from build123d import *

# Parameters (mm, degrees)
SKETCH1_R           = 2.6
SKETCH1_W           = 352.775
SKETCH1_H           = 95.6
BOSS_EXTRUDE1_DEPTH = 3


with BuildPart() as part:
    # Sketch1 → Boss-Extrude1 (new body)
    with BuildSketch(Plane(origin=(0, 0, 0), x_dir=(1, 0, 0), z_dir=(0, 1, 0))):
        with BuildLine():
            Line((4.973e-06, 108.599998007), (4.973e-06, 4.999998007))
            ThreePointArc((4.973e-06, 4.999998007), (1.464471067, 1.464464101), (5.000004973, -1.993e-06))
            Line((5.000004973, -1.993e-06), (365.775004973, -1.993e-06))
            ThreePointArc((365.775004973, -1.993e-06), (369.310538879, 1.464464101), (370.775004973, 4.999998007))
            Line((370.775004973, 4.999998007), (370.775004973, 108.599998007))
            ThreePointArc((370.775004973, 108.599998007), (369.310538879, 112.135531913), (365.775004973, 113.599998007))
            Line((365.775004973, 113.599998007), (5.000004973, 113.599998007))
            ThreePointArc((5.000004973, 113.599998007), (1.464471067, 112.135531913), (4.973e-06, 108.599998007))
        make_face()
        with Locations(Location((5.500004973, 108.099998007, 0), (0, 0, 270))):
            Circle(SKETCH1_R, mode=Mode.SUBTRACT)
        with Locations(Location((5.500004973, 5.499998007, 0), (0, 0, 270))):
            Circle(SKETCH1_R, mode=Mode.SUBTRACT)
        with Locations(Location((365.275004973, 5.499998007, 0), (0, 0, 270))):
            Circle(SKETCH1_R, mode=Mode.SUBTRACT)
        with Locations(Location((365.275004973, 108.099998007, 0), (0, 0, 270))):
            Circle(SKETCH1_R, mode=Mode.SUBTRACT)
        with Locations(Location((35.387504973, 4.499998007, 0), (0, 0, 270))):
            Circle(SKETCH1_R, mode=Mode.SUBTRACT)
        with Locations(Location((135.387504973, 4.499998007, 0), (0, 0, 270))):
            Circle(SKETCH1_R, mode=Mode.SUBTRACT)
        with Locations(Location((335.387504973, 4.499998007, 0), (0, 0, 270))):
            Circle(SKETCH1_R, mode=Mode.SUBTRACT)
        with Locations(Location((235.387504973, 4.499998007, 0), (0, 0, 270))):
            Circle(SKETCH1_R, mode=Mode.SUBTRACT)
        with Locations(Location((35.387504973, 109.099998007, 0), (0, 0, 270))):
            Circle(SKETCH1_R, mode=Mode.SUBTRACT)
        with Locations(Location((135.387504973, 109.099998007, 0), (0, 0, 270))):
            Circle(SKETCH1_R, mode=Mode.SUBTRACT)
        with Locations(Location((335.387504973, 109.099998007, 0), (0, 0, 270))):
            Circle(SKETCH1_R, mode=Mode.SUBTRACT)
        with Locations(Location((235.387504973, 109.099998007, 0), (0, 0, 270))):
            Circle(SKETCH1_R, mode=Mode.SUBTRACT)
        with Locations((185.387504973, 56.799998007)):
            Rectangle(SKETCH1_W, SKETCH1_H, mode=Mode.SUBTRACT)
    extrude(amount=-BOSS_EXTRUDE1_DEPTH)


solid = part.part
Geometry: final body of the model. Coordinates: model frame, mm. Round coordinates to 2 decimals unless told otherwise and drop trailing zeros. Loops run counter-clockwise (first coordinate to the right, second up) from the corner with the lowest first, then second, coordinate; pieces in that order, holes last.
Q1. Material intervals for L1, parallel to Z at x = 336, y = -0.65; L2, parallel to Z at x = 138.5, y = -2.15; L3, parallel to X at y = -0.85, z = -29.5 (3 decimals), sorted ascending.
Q2. Section A-A on x = 278.5. Return loops of the section in (y, z), plus the area to 3 significant figures.
Q3. Section C-C on y = -0.5. State how many separate pieces and enclosed holes the cut face has, plus the area to 3 significant figures.
Q4. Section B-B on z = -31. Return loops of the section in (x, y) (3 decimals).
Q5. Pin query (flat end, axial travel): P1, Ø7, axis at x = 235.39, z = -109.1, coming from the +Y side; P2, Ø4, axis at x = 5.5, z = -108.1, coming from the -Y side. Return the tip coordinate at first contact, or that it passes through.
Evaluation:
1. L1: z = -113.6 to -111.63, -106.57 to -104.6, -9 to -7.03, -1.97 to 0
1. L2: z = -113.6 to -104.6, -9 to 0
1. L3: x = 0 to 9, 361.775 to 370.775
2. outline: (-3, -113.6) - (0, -113.6) - (0, -104.6) - (-3, -104.6) - close; (-3, -9) - (0, -9) - (0, 0) - (-3, 0) - close
2. area: 54.0 mm2
3. separate pieces: 1
3. enclosed holes: 13
3. area: 8,120 mm2
4. outline: (0, -3) - (9, -3) - (9, 0) - (0, 0) - close; (361.775, -3) - (370.775, -3) - (370.775, 0) - (361.775, 0) - close
5. P1: stops at y = 0
5. P2: passes through
